The model under review builds one solid part; all positions refer to its coordinate system, in mm. Coordinates: 2 decimals unless noted, no trailing zeros. Loops run counter-clockwise (first coordinate to the right, second up) from the corner with the lowest first, then second, coordinate; pieces in that order, holes last. Notation, with made-up numbers: (60.25, 87) - (74.25, 87) arc R25 cw to (74.25, 109) - close; hole circle Ø2 at (3.5, 57.25). An arc over 180 degrees is marked (long way). Answer in a Markdown table with one row per item. Add a question column.
(1) We need section A-A on y = 4.25. Write out the cut boundary in (x, z).
(2) For P1, Ø6.5, axis at x = -310, z = 374, coming from the -Y side; P2, Ø4, axis at x = -370.5, z = 270, coming from the -Y side; P3, Ø9.5, axis at y = 17, z = 110, coming from the +X side, all flat-tipped, find the tip position at first contact; note any pin that passes through.
(3) We need section B-B on z = 911. Write out the cut boundary in (x, y).
(4) For line 1 along X through (y, z) = (3.5, 163); line 2 along X through (y, z) = (10.5, -168); line 3 along X through (y, z) = (18.25, 202), list the stretches that pass through material, from the lowest coordinate up.
from build123d import *

# Parameters (mm, degrees)
F0_W     = 130
F0_H     = 1410
F1_DEPTH = 20
F2_W     = 8
F2_H     = 1410
F3_DEPTH = 8
F4_W     = 8
F4_H     = 1460
F5_DEPTH = 12
F6_W     = 8
F6_H     = 1410
F7_DEPTH = 12


with BuildPart() as f1:
    # F0 (on Front) → F1 (new body)
    with BuildSketch(Plane.XZ):
        with Locations((-309.722924, 439.476302)):
            Rectangle(F0_W, F0_H)
    extrude(amount=-F1_DEPTH)

    # F2 (on face) → F3 (cut)
    with BuildSketch(Plane.XZ):
        with Locations((-309.722924, 439.476302)):
            Rectangle(F2_W, F2_H)
    extrude(amount=-F3_DEPTH, mode=Mode.SUBTRACT)

    # F4 (on face) → F5 (cut)
    with BuildSketch(Plane.XZ):
        with Locations((-370.722924, 414.476302)):
            Rectangle(F4_W, F4_H)
    extrude(amount=-F5_DEPTH, mode=Mode.SUBTRACT)

    # F6 (on face) → F7 (cut)
    with BuildSketch(Plane(origin=(0, 20, 0), x_dir=(-1, 0, 0), z_dir=(0, 1, 0))):
        with Locations((248.722924, 439.476302)):
            Rectangle(F6_W, F6_H)
    extrude(amount=-F7_DEPTH, mode=Mode.SUBTRACT)


solid = f1.part
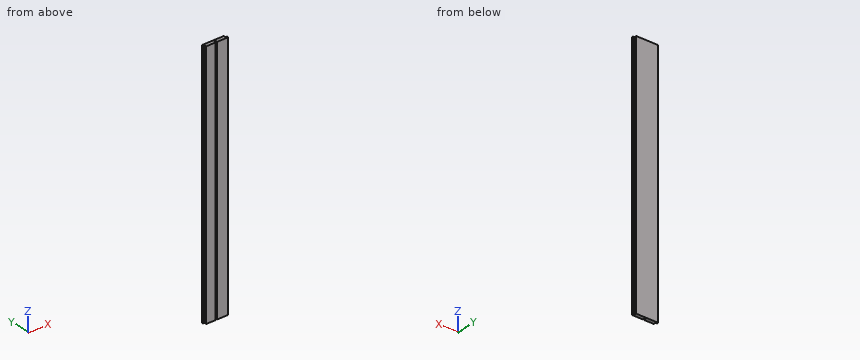
Outcome:
| question | item | result |
|---|---|---|
| 1 | outline | (-366.72, -265.52) - (-313.72, -265.52) - (-313.72, 1144.48) - (-366.72, 1144.48) - close; (-305.72, -265.52) - (-244.72, -265.52) - (-244.72, 1144.48) - (-305.72, 1144.48) - close |
| 2 | P1 | y = 8 |
| 2 | P2 | y = 12 |
| 2 | P3 | x = -252.72 |
| 3 | outline | (-374.72, 12) - (-366.72, 12) - (-366.72, 0) - (-313.72, 0) - (-313.72, 8) - (-305.72, 8) - (-305.72, 0) - (-244.72, 0) - (-244.72, 8) - (-252.72, 8) - (-252.72, 20) - (-374.72, 20) - close |
| 4 | line 1 | -366.72 to -313.72, -305.72 to -244.72 |
| 4 | line 2 | -366.72 to -252.72 |
| 4 | line 3 | -374.72 to -252.72 |
